Source: CAD feature listing. Evaluate the final solid. Frame: model axes, mm. Face numbers are marked on the shaded views. Round coordinates to 2 decimals unless told otherwise and drop trailing zeros. Loops run counter-clockwise (first coordinate to the right, second up) from the corner with the lowest first, then second, coordinate; pieces in that order, holes last. Notation, with made-up numbers: (84, 79) - (115, 79) arc R21 ccw to (115, 98) - close; hole circle Ø2 at (-5, -12). An arc over 180 degrees is marked (long way). One line per question, with ' | ' between items. Start each with the question number.
1. Mould query, pull axis Y, two halves, no side actions, for the marked faces 1 and 2. Classes: pulls with the +Y half, pulls with the -Y half, needs draft (parallel to the pull), parting line crosses it, or undercut.
2. Cut plane B-B (z = 7.5). Return loops of the section in (x, y), then the cut area to 3 significant figures.
3. Cut plane A-A (x = -146.5). Return loops of the section in (y, z).
4. Pin query (flat end, axial travel): pin 1 (0.9 mm diameter, centred on x = -146.5, y = -2, fed in from +Z); pin 2 (1 mm diameter, centred on x = -66.5, y = -1, fed in from -Z); pin 3 (1.5 mm diameter, centred on y = -1.5, z = 20.5, fed in from -X). Return the tip coordinate at first contact, or that it passes through.
5. Ray query, line 1 (Z direction, x = -146.5, y = -2.7); line 2 (X direction, y = -1.3, z = -22); line 3 (X direction, y = -2.1, z = 88). Return the intervals inside material, ascending.
6. Cut plane C-C (x = -22). Return loops of the section in (y, z), then the cut area to 3 significant figures.
```python
from build123d import *

# Parameters (mm, degrees)
F1_DEPTH = 3


with BuildPart() as f1:
    # F0 (on Front) → F1 (new body)
    with BuildSketch(Plane.XZ):
        with BuildLine():
            Line((-100, 71.5043097734), (-100, 30))
            Line((-100, 30), (-68.4474930168, 30))
            ThreePointArc((-68.4474930168, 30), (-89.5290711605, 46.7189281194), (-100, 71.5043097734))
        make_face()
        with BuildLine():
            Line((-68.4474930168, 30), (-100, 30))
            Line((-100, 30), (-100, 23.9479522939))
            ThreePointArc((-100, 23.9479522939), (-77.4009003412, 7.9237058049), (-85.0451834083, -18.7044882255))
            Line((-85.0451834083, -18.7044882255), (-85.0451834083, -30))
            Line((-85.0451834083, -30), (-73.4999999404, -30))
            ThreePointArc((-73.4999999404, -30), (-9.236112237, -22.3609557327), (55.0277754664, -30))
            Line((55.0277754664, -30), (73.458686471, -30))
            Line((73.458686471, -30), (73.458686471, -18.7292341143))
            Line((73.458686471, -18.7292341143), (78.4938633442, -18.7292341143))
            Line((78.4938633442, -18.7292341143), (78.4938633442, -30))
            Line((78.4938633442, -30), (100, -30))
            Line((100, -30), (100, 0))
            Line((100, 0), (100, 30))
            Line((100, 30), (43.509118259, 30))
            ThreePointArc((43.509118259, 30), (17.1951254295, 26.500256647), (-9.3166837469, 25.1592136325))
            Line((-9.3166837469, 25.1592136325), (-9.3166837469, 13.6418417096))
            Line((-9.3166837469, 13.6418417096), (-15.6216910109, 13.6418417096))
            Line((-15.6216910109, 13.6418417096), (-15.6216910109, 25.1592136325))
            ThreePointArc((-15.6216910109, 25.1592136325), (-42.1335001872, 26.500256647), (-68.4474930168, 30))
        make_face()
        with BuildLine():
            Line((-100, 23.9479522939), (-100, 30))
            Line((-100, 30), (-100, 71.5043097734))
            Line((-100, 71.5043097734), (-124.3806779385, 71.5043097734))
            Line((-124.3806779385, 71.5043097734), (-124.3806779385, 44.8159986225))
            Line((-124.3806779385, 44.8159986225), (-124.3806779385, 39.189517498))
            Line((-124.3806779385, 39.189517498), (-124.3806779385, 0))
            Line((-124.3806779385, 0), (-123.9479522939, 0))
            ThreePointArc((-123.9479522939, 0), (-116.9337594626, 16.9337594626), (-100, 23.9479522939))
        make_face()
        with BuildLine():
            ThreePointArc((-85.0451834083, -18.7044882255), (-77.4009003412, 7.9237058049), (-100, 23.9479522939))
            Line((-100, 23.9479522939), (-100, 0))
            Line((-100, 0), (-100, -23.9479522939))
            ThreePointArc((-100, -23.9479522939), (-93.7566918243, -23.119808003), (-87.9451834083, -20.6926512562))
            Line((-87.9451834083, -20.6926512562), (-87.9451834083, -18.0708928406))
            Line((-87.9451834083, -18.0708928406), (-85.0451834083, -18.0708928406))
            Line((-85.0451834083, -18.0708928406), (-85.0451834083, -18.7044882255))
        make_face()
        with BuildLine():
            Line((-100, 0), (-100, 23.9479522939))
            ThreePointArc((-100, 23.9479522939), (-116.9337594626, 16.9337594626), (-123.9479522939, 0))
            Line((-123.9479522939, 0), (-100, 0))
        make_face()
        with BuildLine():
            Line((-124.3806779385, 71.5043097734), (-100, 71.5043097734))
            ThreePointArc((-100, 71.5043097734), (-107.5768900996, 87.9325587369), (-124.3806779385, 94.6354940534))
            Line((-124.3806779385, 94.6354940534), (-124.3806779385, 71.5043097734))
        make_face()
        with BuildLine():
            Line((-100, -23.9479522939), (-100, 0))
            Line((-100, 0), (-123.9479522939, 0))
            ThreePointArc((-123.9479522939, 0), (-123.561080085, -4.2871813932), (-122.4129630745, -8.4358464478))
            ThreePointArc((-122.4129630745, -8.4358464478), (-121.2500665042, -10.9208672377), (-119.9064756979, -13.3130253647))
            ThreePointArc((-119.9064756979, -13.3130253647), (-111.2846072761, -21.1225485606), (-100, -23.9479522939))
        make_face()
        Polygon((-124.3806779385, 44.8159986225), (-124.3806779385, 71.5043097734), (-124.3806779385, 94.6354940534), (-154.4115646049, 94.6354940534), (-154.4115646049, 81.2257463379), (-124.6924658106, 81.2257463379), (-124.6924658106, 58.2257463379), (-154.4115646049, 58.2257463379), (-154.4115646049, 44.8159986225), (-140.5599779571, 44.8159986225), align=None)
        with BuildLine():
            ThreePointArc((-87.9451834083, -20.6926512562), (-93.7566918243, -23.119808003), (-100, -23.9479522939))
            Line((-100, -23.9479522939), (-100, -27))
            ThreePointArc((-100, -27), (-99.5920709422, -28.5103536773), (-98.4792211797, -29.6099625862))
            ThreePointArc((-98.4792211797, -29.6099625862), (-97.7416237075, -29.812616064), (-97, -30))
            Line((-97, -30), (-87.9451834083, -30))
            Line((-87.9451834083, -30), (-87.9451834083, -20.6926512562))
        make_face()
        with BuildLine():
            Line((-100, -27), (-100, -23.9479522939))
            ThreePointArc((-100, -23.9479522939), (-111.2846072761, -21.1225485606), (-119.9064756979, -13.3130253647))
            ThreePointArc((-119.9064756979, -13.3130253647), (-110.7252490766, -23.4762982325), (-98.4792211797, -29.6099625862))
            ThreePointArc((-98.4792211797, -29.6099625862), (-99.5920709422, -28.5103536773), (-100, -27))
        make_face()
        with BuildLine():
            ThreePointArc((-119.9064756979, -13.3130253647), (-121.2500665042, -10.9208672377), (-122.4129630745, -8.4358464478))
            ThreePointArc((-122.4129630745, -8.4358464478), (-121.2997756573, -10.946413843), (-119.9064756979, -13.3130253647))
        make_face()
        with BuildLine():
            Line((-124.3806779385, 39.189517498), (-124.3806779385, 44.8159986225))
            Line((-124.3806779385, 44.8159986225), (-140.5599779571, 44.8159986225))
            ThreePointArc((-140.5599779571, 44.8159986225), (-132.2111646691, 42.7479983529), (-124.3806779385, 39.189517498))
        make_face()
        with BuildLine():
            Line((-154.4115646049, 81.2257463379), (-154.4115646049, 94.6354940534))
            ThreePointArc((-154.4115646049, 94.6354940534), (-163.4199195991, 91.0594551964), (-167.5229668617, 82.2785943747))
            Line((-167.5229668617, 82.2785943747), (-154.4115646049, 81.2257463379))
        make_face()
        with BuildLine():
            ThreePointArc((-97, -30), (-97.7416237075, -29.812616064), (-98.4792211797, -29.6099625862))
            ThreePointArc((-98.4792211797, -29.6099625862), (-97.7648896134, -29.9008522678), (-97, -30))
        make_face()
        Polygon((-167.5229668617, 55.4901845753), (-154.4115646049, 44.8159986225), (-154.4115646049, 58.2257463379), align=None)
        with BuildLine():
            ThreePointArc((100, 108.6442619568), (82.0137314179, 61.9528751155), (43.509118259, 30))
            Line((43.509118259, 30), (100, 30))
            Line((100, 30), (100, 108.6442619568))
        make_face()
        with BuildLine():
            ThreePointArc((100.2573479135, 108.64405), (100.1286740004, 108.6442089676), (100, 108.6442619568))
            Line((100, 108.6442619568), (100, 30))
            Line((100, 30), (100, 0))
            Line((100, 0), (128.8781613111, 0))
            Line((128.8781613111, 0), (128.8781613111, 80.0234485584))
            ThreePointArc((128.8781613111, 80.0234485584), (108.6402650122, 88.4062157818), (100.2573479135, 108.64405))
        make_face()
        with BuildLine():
            Line((100.2573479127, 108.6442619568), (100, 108.6442619568))
            ThreePointArc((100, 108.6442619568), (100.1286740004, 108.6442089676), (100.2573479135, 108.64405))
            ThreePointArc((100.2573479135, 108.64405), (100.2573479129, 108.6441559784), (100.2573479127, 108.6442619568))
        make_face()
        with BuildLine():
            ThreePointArc((142.8596985833, 133.6175992408), (114.4042539206, 133.3354944988), (100.2573479127, 108.6442619568))
            Line((100.2573479127, 108.6442619568), (128.8781613111, 108.6442619568))
            Line((128.8781613111, 108.6442619568), (142.8596985833, 133.6175992408))
        make_face()
        with BuildLine():
            Line((128.8781613111, 108.6442619568), (100.2573479127, 108.6442619568))
            ThreePointArc((100.2573479127, 108.6442619568), (100.2573479129, 108.6441559784), (100.2573479135, 108.64405))
            ThreePointArc((100.2573479135, 108.64405), (114.6298030847, 107.9577659942), (128.8781613111, 105.9520887429))
            Line((128.8781613111, 105.9520887429), (128.8781613111, 108.6442619568))
        make_face()
        with BuildLine():
            ThreePointArc((128.8781613111, 105.9520887429), (114.6298030847, 107.9577659942), (100.2573479135, 108.64405))
            ThreePointArc((100.2573479135, 108.64405), (108.6402650122, 88.4062157818), (128.8781613111, 80.0234485584))
            Line((128.8781613111, 80.0234485584), (128.8781613111, 105.9520887429))
        make_face()
        with BuildLine():
            Line((128.8781613111, 0), (100, 0))
            Line((100, 0), (100, -30))
            ThreePointArc((100, -30), (117.2918939431, -17.7461334103), (128.8781613111, 0))
        make_face()
    extrude(amount=F1_DEPTH)


solid = f1.part
```
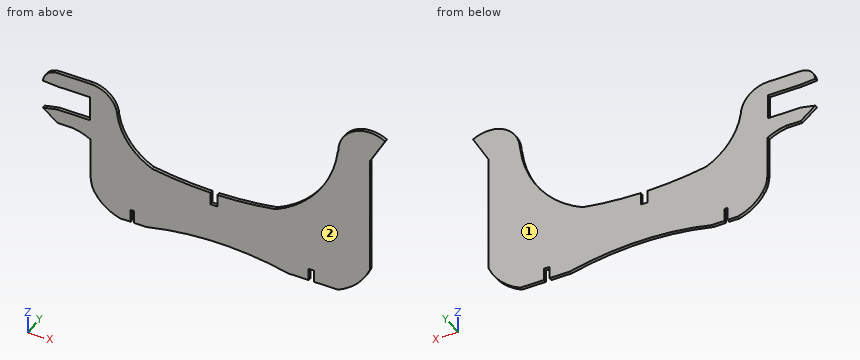
Answers follow:
1) face 1: pulls with the +Y half | face 2: pulls with the -Y half
2) outline: (-124.38, -3) - (128.88, -3) - (128.88, 0) - (-124.38, 0) - close | area: 760 mm2
3) outline: (-3, 44.82) - (0, 44.82) - (0, 58.23) - (-3, 58.23) - close; (-3, 81.23) - (0, 81.23) - (0, 94.64) - (-3, 94.64) - close
4) pin 1: stops at z = 94.64 | pin 2: stops at z = -28.52 | pin 3: stops at x = -124.38
5) line 1: z = 44.82 to 58.23, 81.23 to 94.64 | line 2: x = -112.54 to -87.95, -85.05 to 73.46, 78.49 to 112.72 | line 3: x = -165.83 to -107.65, 95.4 to 128.88
6) outline: (-3, -22.66) - (0, -22.66) - (0, 25.28) - (-3, 25.28) - close | area: 144 mm2
